from build123d import *

# Parameters (mm, degrees)
F1_DEPTH = 5
F2_R     = 1
F3_DEPTH = 5.001
F5_DEPTH = 5


with BuildPart() as f1:
    # F0 (on Top) → F1 (new body)
    with BuildSketch(Plane.XY):
        with BuildLine():
            ThreePointArc((7.4206173165, -1.0883191822), (7.4801280027, -0.5456052265), (7.5, 0))
            ThreePointArc((7.5, 0), (7.4801280027, 0.5456052265), (7.4206173165, 1.0883191822))
            ThreePointArc((7.4206173165, 1.0883191822), (7.355889603, 1.4631774151), (7.2722381774, 1.8342714877))
            ThreePointArc((7.2722381774, 1.8342714877), (6.9290964938, 2.8701257427), (6.4392747372, 3.8452231222))
            ThreePointArc((6.4392747372, 3.8452231222), (6.2360220923, 4.1667767476), (6.0167266989, 4.4776109513))
            ThreePointArc((6.0167266989, 4.4776109513), (5.3033008589, 5.3033008589), (4.4776109513, 6.0167266989))
            ThreePointArc((4.4776109513, 6.0167266989), (4.1667767476, 6.2360220923), (3.8452231222, 6.4392747372))
            ThreePointArc((3.8452231222, 6.4392747372), (2.8701257427, 6.9290964938), (1.8342714877, 7.2722381774))
            ThreePointArc((1.8342714877, 7.2722381774), (1.4631774151, 7.355889603), (1.0883191822, 7.4206173165))
            ThreePointArc((1.0883191822, 7.4206173165), (0, 7.5), (-1.0883191822, 7.4206173165))
            ThreePointArc((-1.0883191822, 7.4206173165), (-1.4631774151, 7.355889603), (-1.8342714877, 7.2722381774))
            ThreePointArc((-1.8342714877, 7.2722381774), (-2.8701257427, 6.9290964938), (-3.8452231222, 6.4392747372))
            ThreePointArc((-3.8452231222, 6.4392747372), (-4.1667767476, 6.2360220923), (-4.4776109513, 6.0167266989))
            ThreePointArc((-4.4776109513, 6.0167266989), (-5.3033008589, 5.3033008589), (-6.0167266989, 4.4776109513))
            ThreePointArc((-6.0167266989, 4.4776109513), (-6.2360220923, 4.1667767476), (-6.4392747372, 3.8452231222))
            ThreePointArc((-6.4392747372, 3.8452231222), (-6.9290964938, 2.8701257427), (-7.2722381774, 1.8342714877))
            ThreePointArc((-7.2722381774, 1.8342714877), (-7.355889603, 1.4631774151), (-7.4206173165, 1.0883191822))
            ThreePointArc((-7.4206173165, 1.0883191822), (-7.5, 0), (-7.4206173165, -1.0883191822))
            ThreePointArc((-7.4206173165, -1.0883191822), (-7.355889603, -1.4631774151), (-7.2722381774, -1.8342714877))
            ThreePointArc((-7.2722381774, -1.8342714877), (-6.9290964938, -2.8701257427), (-6.4392747372, -3.8452231222))
            ThreePointArc((-6.4392747372, -3.8452231222), (-6.2360220923, -4.1667767476), (-6.0167266989, -4.4776109513))
            ThreePointArc((-6.0167266989, -4.4776109513), (-5.3033008589, -5.3033008589), (-4.4776109513, -6.0167266989))
            ThreePointArc((-4.4776109513, -6.0167266989), (-4.1667767476, -6.2360220923), (-3.8452231222, -6.4392747372))
            ThreePointArc((-3.8452231222, -6.4392747372), (-2.8701257427, -6.9290964938), (-1.8342714877, -7.2722381774))
            ThreePointArc((-1.8342714877, -7.2722381774), (-1.4631774151, -7.355889603), (-1.0883191822, -7.4206173165))
            ThreePointArc((-1.0883191822, -7.4206173165), (0, -7.5), (1.0883191822, -7.4206173165))
            ThreePointArc((1.0883191822, -7.4206173165), (1.4631774151, -7.355889603), (1.8342714877, -7.2722381774))
            ThreePointArc((1.8342714877, -7.2722381774), (2.8701257427, -6.9290964938), (3.8452231222, -6.4392747372))
            ThreePointArc((3.8452231222, -6.4392747372), (4.1667767476, -6.2360220923), (4.4776109513, -6.0167266989))
            ThreePointArc((4.4776109513, -6.0167266989), (5.3033008589, -5.3033008589), (6.0167266989, -4.4776109513))
            ThreePointArc((6.0167266989, -4.4776109513), (6.2360220923, -4.1667767476), (6.4392747372, -3.8452231222))
            ThreePointArc((6.4392747372, -3.8452231222), (6.9290964938, -2.8701257427), (7.2722381774, -1.8342714877))
            ThreePointArc((7.2722381774, -1.8342714877), (7.355889603, -1.4631774151), (7.4206173165, -1.0883191822))
        make_face()
        with BuildLine():
            ThreePointArc((7.4206173165, 1.0883191822), (7.4801280027, 0.5456052265), (7.5, 0))
            ThreePointArc((7.5, 0), (7.4801280027, -0.5456052265), (7.4206173165, -1.0883191822))
            ThreePointArc((7.4206173165, -1.0883191822), (8.5043518229, -0.9498278009), (9.5, -0.5))
            Line((9.5, -0.5), (9.5, 0))
            Line((9.5, 0), (9.5, 0.5))
            ThreePointArc((9.5, 0.5), (8.5043518229, 0.9498278009), (7.4206173165, 1.0883191822))
        make_face()
        with BuildLine():
            ThreePointArc((6.4392747372, 3.8452231222), (6.9290964938, 2.8701257427), (7.2722381774, 1.8342714877))
            ThreePointArc((7.2722381774, 1.8342714877), (8.2204799494, 2.376948081), (8.968197275, 3.1735528412))
            Line((8.968197275, 3.1735528412), (8.7768555589, 3.6354926075))
            Line((8.7768555589, 3.6354926075), (8.5855138427, 4.0974323737))
            ThreePointArc((8.5855138427, 4.0974323737), (7.4935132234, 4.1320010103), (6.4392747372, 3.8452231222))
        make_face()
        with BuildLine():
            ThreePointArc((8.968197275, -3.1735528412), (8.2204799494, -2.376948081), (7.2722381774, -1.8342714877))
            ThreePointArc((7.2722381774, -1.8342714877), (6.9290964938, -2.8701257427), (6.4392747372, -3.8452231222))
            ThreePointArc((6.4392747372, -3.8452231222), (7.4935132234, -4.1320010103), (8.5855138427, -4.0974323737))
            Line((8.5855138427, -4.0974323737), (8.7768555589, -3.6354926075))
            Line((8.7768555589, -3.6354926075), (8.968197275, -3.1735528412))
        make_face()
        with BuildLine():
            ThreePointArc((4.4776109513, 6.0167266989), (5.3033008589, 5.3033008589), (6.0167266989, 4.4776109513))
            ThreePointArc((6.0167266989, 4.4776109513), (6.6851145225, 5.3418551646), (7.0710678119, 6.3639610307))
            Line((7.0710678119, 6.3639610307), (6.7175144213, 6.7175144213))
            Line((6.7175144213, 6.7175144213), (6.3639610307, 7.0710678119))
            ThreePointArc((6.3639610307, 7.0710678119), (5.3418551646, 6.6851145225), (4.4776109513, 6.0167266989))
        make_face()
        with BuildLine():
            ThreePointArc((7.0710678119, -6.3639610307), (6.6851145225, -5.3418551646), (6.0167266989, -4.4776109513))
            ThreePointArc((6.0167266989, -4.4776109513), (5.3033008589, -5.3033008589), (4.4776109513, -6.0167266989))
            ThreePointArc((4.4776109513, -6.0167266989), (5.3418551646, -6.6851145225), (6.3639610307, -7.0710678119))
            Line((6.3639610307, -7.0710678119), (6.7175144213, -6.7175144213))
            Line((6.7175144213, -6.7175144213), (7.0710678119, -6.3639610307))
        make_face()
        with BuildLine():
            ThreePointArc((1.8342714877, 7.2722381774), (2.8701257427, 6.9290964938), (3.8452231222, 6.4392747372))
            ThreePointArc((3.8452231222, 6.4392747372), (4.1320010103, 7.4935132234), (4.0974323737, 8.5855138427))
            Line((4.0974323737, 8.5855138427), (3.6354926075, 8.7768555589))
            Line((3.6354926075, 8.7768555589), (3.1735528412, 8.968197275))
            ThreePointArc((3.1735528412, 8.968197275), (2.376948081, 8.2204799494), (1.8342714877, 7.2722381774))
        make_face()
        with BuildLine():
            ThreePointArc((4.0974323737, -8.5855138427), (4.1320010103, -7.4935132234), (3.8452231222, -6.4392747372))
            ThreePointArc((3.8452231222, -6.4392747372), (2.8701257427, -6.9290964938), (1.8342714877, -7.2722381774))
            ThreePointArc((1.8342714877, -7.2722381774), (2.376948081, -8.2204799494), (3.1735528412, -8.968197275))
            Line((3.1735528412, -8.968197275), (3.6354926075, -8.7768555589))
            Line((3.6354926075, -8.7768555589), (4.0974323737, -8.5855138427))
        make_face()
        with BuildLine():
            ThreePointArc((-1.0883191822, 7.4206173165), (0, 7.5), (1.0883191822, 7.4206173165))
            ThreePointArc((1.0883191822, 7.4206173165), (0.9498278009, 8.5043518229), (0.5, 9.5))
            Line((0.5, 9.5), (0, 9.5))
            Line((0, 9.5), (-0.5, 9.5))
            ThreePointArc((-0.5, 9.5), (-0.9498278009, 8.5043518229), (-1.0883191822, 7.4206173165))
        make_face()
        with BuildLine():
            ThreePointArc((0.5, -9.5), (0.9498278009, -8.5043518229), (1.0883191822, -7.4206173165))
            ThreePointArc((1.0883191822, -7.4206173165), (0, -7.5), (-1.0883191822, -7.4206173165))
            ThreePointArc((-1.0883191822, -7.4206173165), (-0.9498278009, -8.5043518229), (-0.5, -9.5))
            Line((-0.5, -9.5), (0, -9.5))
            Line((0, -9.5), (0.5, -9.5))
        make_face()
        with BuildLine():
            ThreePointArc((-3.8452231222, 6.4392747372), (-2.8701257427, 6.9290964938), (-1.8342714877, 7.2722381774))
            ThreePointArc((-1.8342714877, 7.2722381774), (-2.376948081, 8.2204799494), (-3.1735528412, 8.968197275))
            Line((-3.1735528412, 8.968197275), (-3.6354926075, 8.7768555589))
            Line((-3.6354926075, 8.7768555589), (-4.0974323737, 8.5855138427))
            ThreePointArc((-4.0974323737, 8.5855138427), (-4.1320010103, 7.4935132234), (-3.8452231222, 6.4392747372))
        make_face()
        with BuildLine():
            ThreePointArc((-3.1735528412, -8.968197275), (-2.376948081, -8.2204799494), (-1.8342714877, -7.2722381774))
            ThreePointArc((-1.8342714877, -7.2722381774), (-2.8701257427, -6.9290964938), (-3.8452231222, -6.4392747372))
            ThreePointArc((-3.8452231222, -6.4392747372), (-4.1320010103, -7.4935132234), (-4.0974323737, -8.5855138427))
            Line((-4.0974323737, -8.5855138427), (-3.6354926075, -8.7768555589))
            Line((-3.6354926075, -8.7768555589), (-3.1735528412, -8.968197275))
        make_face()
        with BuildLine():
            ThreePointArc((-6.0167266989, 4.4776109513), (-5.3033008589, 5.3033008589), (-4.4776109513, 6.0167266989))
            ThreePointArc((-4.4776109513, 6.0167266989), (-5.3418551646, 6.6851145225), (-6.3639610307, 7.0710678119))
            Line((-6.3639610307, 7.0710678119), (-6.7175144213, 6.7175144213))
            Line((-6.7175144213, 6.7175144213), (-7.0710678119, 6.3639610307))
            ThreePointArc((-7.0710678119, 6.3639610307), (-6.6851145225, 5.3418551646), (-6.0167266989, 4.4776109513))
        make_face()
        with BuildLine():
            ThreePointArc((-6.3639610307, -7.0710678119), (-5.3418551646, -6.6851145225), (-4.4776109513, -6.0167266989))
            ThreePointArc((-4.4776109513, -6.0167266989), (-5.3033008589, -5.3033008589), (-6.0167266989, -4.4776109513))
            ThreePointArc((-6.0167266989, -4.4776109513), (-6.6851145225, -5.3418551646), (-7.0710678119, -6.3639610307))
            Line((-7.0710678119, -6.3639610307), (-6.7175144213, -6.7175144213))
            Line((-6.7175144213, -6.7175144213), (-6.3639610307, -7.0710678119))
        make_face()
        with BuildLine():
            ThreePointArc((-7.2722381774, 1.8342714877), (-6.9290964938, 2.8701257427), (-6.4392747372, 3.8452231222))
            ThreePointArc((-6.4392747372, 3.8452231222), (-7.4935132234, 4.1320010103), (-8.5855138427, 4.0974323737))
            Line((-8.5855138427, 4.0974323737), (-8.7768555589, 3.6354926075))
            Line((-8.7768555589, 3.6354926075), (-8.968197275, 3.1735528412))
            ThreePointArc((-8.968197275, 3.1735528412), (-8.2204799494, 2.376948081), (-7.2722381774, 1.8342714877))
        make_face()
        with BuildLine():
            ThreePointArc((-8.5855138427, -4.0974323737), (-7.4935132234, -4.1320010103), (-6.4392747372, -3.8452231222))
            ThreePointArc((-6.4392747372, -3.8452231222), (-6.9290964938, -2.8701257427), (-7.2722381774, -1.8342714877))
            ThreePointArc((-7.2722381774, -1.8342714877), (-8.2204799494, -2.376948081), (-8.968197275, -3.1735528412))
            Line((-8.968197275, -3.1735528412), (-8.7768555589, -3.6354926075))
            Line((-8.7768555589, -3.6354926075), (-8.5855138427, -4.0974323737))
        make_face()
        with BuildLine():
            ThreePointArc((-7.4206173165, -1.0883191822), (-7.5, 0), (-7.4206173165, 1.0883191822))
            ThreePointArc((-7.4206173165, 1.0883191822), (-8.5043518229, 0.9498278009), (-9.5, 0.5))
            Line((-9.5, 0.5), (-9.5, 0))
            Line((-9.5, 0), (-9.5, -0.5))
            ThreePointArc((-9.5, -0.5), (-8.5043518229, -0.9498278009), (-7.4206173165, -1.0883191822))
        make_face()
    extrude(amount=F1_DEPTH)

    # F2 (on face) → F3 (cut, through all)
    with BuildSketch(Plane.XY.offset(5)):
        Circle(F2_R)
    extrude(amount=-F3_DEPTH, mode=Mode.SUBTRACT)

    # F4 (on Top) → F5 (join, through all)
    with BuildSketch(Plane.XY):
        with BuildLine():
            add(Edge.make_bspline(
                [(0, 68), (10, 68), (26.5357793377, 69.6195584207), (35.7921763751, 15.3144879989), (16.2360220923, -4.1667767476), (6.2360220923, -4.1667767476)],
                knots=[0, 0, 0, 0, 0.2773691883, 0.6738677823, 1, 1, 1, 1], degree=3))
            Line((0, 68), (0, 60))
            add(Edge.make_bspline(
                [(0, 60), (10, 60), (20.2377735158, 60.6776605511), (25.2912821546, 26.6920800115), (16.2360220923, 4.1667767476), (6.2360220923, 4.1667767476)],
                knots=[0, 0, 0, 0, 0.28371621, 0.6494672366, 1, 1, 1, 1], degree=3))
            Line((6.2360220923, 4.1667767476), (6.2360220923, -4.1667767476))
        make_face()
    extrude(amount=F5_DEPTH)


solid = f1.part
Input: part model. Units: mm. Frame: model coordinates. A direction names the side the tool comes from. Give positions to 0.01 mm unless a question says otherwise; leave off trailing zeros. Answer as a JSON object with one key per item and string values. Group by question number.
Q1. Line query: probe 1 along Y at (x, z) = (9.5, 3.25); probe 2 along Y at (x, z) = (11, 2.3); probe 3 along X at (y, z) = (39.5, 1.15). Output: solid intervals per line, ascending.
Q2. First-contact query: pin 1 Ø1 at (y, z) = (10.5, 4) entering from -X; pin 2 Ø1.5 at (x, z) = (17.5, 3) entering from -Y; pin 3 Ø2 at (x, z) = (18.5, 1) entering from +Y; pin 4 Ø10 at (x, y) = (20.5, 53) entering from -Z. Flat tips, straight axial feed; report the tip coordinate or a pass-through.
Q3. Mould query, pull axis X, two halves, no side actions, for faces 5 (the face through (-4.134, 7.509, 2.465)), 6 (the face through (6.693, -5.355, 2.465)), 7 (the face through (-2.37, 8.21, 2.46)), 8 (the face through (-6.68, -5.33, 2.46)). Classes: pulls with the +X half, pulls with the -X half, needs draft (parallel to the pull), parting line crosses it, or undercut.
Q4. Set-up query: faces 1 (the face through (5.355, 6.693, 2.465)), 2 (the face through (5.33, -6.68, 2.46)), 3 (the face through (-8.233, 2.386, 2.465)), 4 (the face through (23, 24, 0)). Return all of +Z, -Z, +X, -X, +Y, -Y with unobstructed straight access to the full face (end or side cutting, diameter ignored); none if empty.
Results:
{
 "1": {"probe 1": "-3.85 to 4.6, 59.85 to 67.93", "probe 2": "-3.49 to 5.13, 59.7 to 67.83", "probe 3": "22.39 to 29.94"},
 "2": {"pin 1": "x = 16.66", "pin 2": "y = -0.72", "pin 3": "y = 66.22", "pin 4": "z = 0"},
 "3": {"face 5": "undercut", "face 6": "pulls with the +X half", "face 7": "undercut", "face 8": "pulls with the -X half"},
 "4": {"face 1": "+Z, -Z", "face 2": "+Z, -Z, -Y", "face 3": "+Z, -Z, -X", "face 4": "-Z, +X, -X, +Y, -Y"}
}
